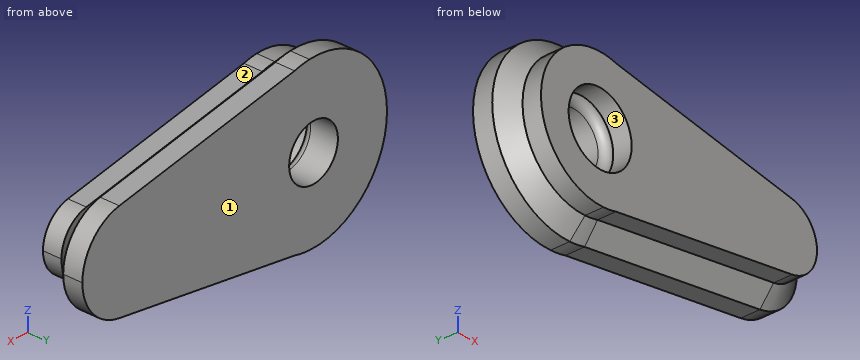
```python
from build123d import *

# Parameters (mm, degrees)
F0_R     = 8.6726561419
F1_DEPTH = 11.176
F2_R     = 2.54
F3_SIZE  = 5.08
F4_DEPTH = 5.842


with BuildPart() as f1:
    # F0 (on Front) → F1 (new body)
    with BuildSketch(Plane.XZ):
        with BuildLine():
            ThreePointArc((-3.7094716517, 32.7638350621), (-6.3317193926, 33.3185695674), (-8.9969745918, 33.6019920596))
            Line((-8.9969745918, 33.6019920596), (-3.7094716517, 32.7638350621))
        make_face()
        with BuildLine():
            Line((-3.7094716517, -17.7854802654), (-8.9969745918, -18.6236372628))
            ThreePointArc((-8.9969745918, -18.6236372628), (-6.3317193926, -18.3402147707), (-3.7094716517, -17.7854802654))
        make_face()
        with BuildLine():
            Line((58.6809857184, 22.8739117825), (-3.7094716517, 32.7638350621))
            ThreePointArc((-3.7094716517, 32.7638350621), (10.3052007911, 23.4307705289), (15.7257861582, 7.4891773984))
            ThreePointArc((15.7257861582, 7.4891773984), (10.3052007911, -8.4524157321), (-3.7094716517, -17.7854802654))
            Line((-3.7094716517, -17.7854802654), (58.6809857184, -7.8955569857))
            ThreePointArc((58.6809857184, -7.8955569857), (40.6654246701, 7.4891773984), (58.6809857184, 22.8739117825))
        make_face()
        with BuildLine():
            ThreePointArc((71.819075142, 7.4891773984), (68.087612838, 17.6047525893), (58.6809857184, 22.8739117825))
            ThreePointArc((58.6809857184, 22.8739117825), (40.6654246701, 7.4891773984), (58.6809857184, -7.8955569857))
            ThreePointArc((58.6809857184, -7.8955569857), (68.087612838, -2.6263977925), (71.819075142, 7.4891773984))
        make_face()
        with BuildLine():
            Line((-3.7094716517, 32.7638350621), (-8.9969745918, 33.6019920596))
            ThreePointArc((-8.9969745918, 33.6019920596), (-36.5779998836, 7.4891773984), (-8.9969745918, -18.6236372628))
            Line((-8.9969745918, -18.6236372628), (-3.7094716517, -17.7854802654))
            ThreePointArc((-3.7094716517, -17.7854802654), (10.3052007911, -8.4524157321), (15.7257861582, 7.4891773984))
            ThreePointArc((15.7257861582, 7.4891773984), (10.3052007911, 23.4307705289), (-3.7094716517, 32.7638350621))
        make_face()
        with Locations((-10.4261068627, 7.4891773984)):
            Circle(F0_R, mode=Mode.SUBTRACT)
    extrude(amount=F1_DEPTH)

    # F2
    f2_edges = [f1.edges().sort_by_distance(p)[0] for p in [
        (-19.098763, -11.176, 7.489177),
    ]]
    fillet(f2_edges, radius=F2_R)

    # F3
    f3_edges = [f1.edges().sort_by_distance(p)[0] for p in [
        (27.485757, -11.176, -12.840519),
        (-21.638763, -11.176, 7.489177),
        (-36.578, -11.176, 7.489177),
        (71.819075, -11.176, 7.489177),
        (27.485757, -11.176, 27.818873),
    ]]
    chamfer(f3_edges, length=F3_SIZE)

    # F4 (add): a face of the model
    f4_faces = [f1.faces().sort_by_distance(p)[0] for p in [
        (16.1234060629, -11.176, 7.4891773984),
    ]]
    extrude(f4_faces, amount=F4_DEPTH)


solid = f1.part
```
Geometry check sheet. Reference: the model listing, model coordinates, mm. Face numbers are marked on the shaded views. A direction names the side the tool comes from. Coordinates: 2 decimals unless noted, no trailing zeros. Order: outer loops, then holes, each group sorted by start corner. A loop starts at its lowest first (then second) coordinate and runs counter-clockwise, first axis right, second up.
Q1. Depth check by flat-ended pin: pin 1 Ø5 at (x, z) = (58.5, 27.5) entering from -Y; pin 2 Ø2 at (x, y) = (39, -11.5) entering from +Z; pin 3 Ø2 at (x, y) = (-17.5, -8.5) entering from +Z; pin 4 Ø6 at (x, z) = (58, 24.5) entering from -Y. Enter the tip coordinate at first touch or a pass-through.
Reply:
pin 1: passes through
pin 2: stops at z = 21.55
pin 3: stops at z = 31.24
pin 4: stops at y = -7.6
Q2. Thickness scan on probe 1 along X at (y, z) = (-1.5, 7); probe 2 along X at (y, z) = (-12.5, 5.5); probe 3 along Z at (x, y) = (61, -9.5). Record the ranges inside material, lowest first.
Reply:
probe 1: x = -36.57 to -19.08, -1.77 to 71.81
probe 2: x = -31.4 to -21.46, 0.61 to 66.55
probe 3: z = -3.72 to 18.69
Q3. Sectioned sample at A-A on y = -12.25. Record the cut outline in (x, z), and give its area (3 significant figures).
Reply:
outline: (-4.78, -12.81) - (57.89, -2.88) arc R10.5 ccw to (57.89, 17.86) - (-4.78, 27.79) arc R21.07 ccw (long way) to start; hole circle Ø22.43 at (-10.43, 7.49)
area: 2,600 mm2
Q4. Tool access check on the marked faces 1, 2 and 3. Record the directions out of +Z, -Z, +X, -X, +Y, -Y that give a thin tool (end or side, any length) a straight path to the whole face; none if there is none.
Reply:
face 1: +Z, -Z, +X, -X, +Y
face 2: +Z, +X, -Y
face 3: -Y
Q5. Sectioned sample at D-D on x = 2. Record the cut outline in (y, z), and give its area (3 significant figures).
Reply:
outline: (-17.02, -11.74) - (-11.18, -11.74) - (-6.1, -16.88) - (0, -16.88) - (0, 31.86) - (-6.1, 31.86) - (-11.18, 26.72) - (-17.02, 26.72) - close
area: 743 mm2
Q6. Sectioned sample at C-C on y = -3.5. Record the cut outline in (x, z).
Reply:
outline: (-3.71, -17.79) - (58.68, -7.9) arc R15.58 ccw to (58.68, 22.87) - (-3.71, 32.76) arc R26.15 ccw (long way) to start; hole circle Ø17.35 at (-10.43, 7.49)
Q7. Sectioned sample at B-B on x = 40. Record the cut outline in (y, z), and give its area (3 significant figures).
Reply:
outline: (-17.02, -5.71) - (-11.18, -5.71) - (-6.1, -10.86) - (0, -10.86) - (0, 25.84) - (-6.1, 25.84) - (-11.18, 20.69) - (-17.02, 20.69) - close
area: 538 mm2
